```python
from build123d import *

# Parameters (mm, degrees)
BOSS_EXTRUDE1_DEPTH = 38.1
CUT_EXTRUDE1_DEPTH  = 98.457965419
SHELL1_START        = -37.25333418
SHELL1_DEPTH        = 74.50666836
FILLET1_R           = 17.78
SKETCH3_W           = 12.7
SKETCH3_H           = 13.97
CUT_EXTRUDE2_DEPTH  = 2.54


# Read off the part's stored shape, not the designer's step: Shell1
with BuildPart() as part:
    # Sketch1 → Boss-Extrude1 (new, symmetric)
    with BuildSketch(Plane.XY):
        Polygon((-33.198119966, 25.4), (-33.198119966, -25.4), (33.198119966, -50.887128572), (33.198119966, -0.087128572), align=None)
    extrude(amount=BOSS_EXTRUDE1_DEPTH, both=True)

    # Sketch2 → Cut-Extrude1 (cut, through all)
    with BuildSketch(Plane.XY.offset(38.1)):
        Polygon((16.599059983, -44.515346429), (33.198119966, -33.107128572), (33.198119966, -50.887128572), align=None)
        Polygon((-16.599059983, 19.028217857), (-33.198119966, 25.4), (-33.198119966, 7.62), align=None)
    extrude(amount=-CUT_EXTRUDE1_DEPTH, mode=Mode.SUBTRACT)

    # Shell1 outline → Shell1 (cut)
    with BuildSketch(Plane.XY.offset(SHELL1_START)):
        Polygon((-32.351454146, 7.174547563), (-32.351454146, -24.818102704), (16.486612201, -43.565279915), (31.928119966, -32.952625656), (31.928119966, 0.400378753), (-15.639946381, 18.66004864), align=None)
    extrude(amount=SHELL1_DEPTH, mode=Mode.SUBTRACT)

    # Fillet1
    # the kernel refuses this fillet: 17.78 mm, written as the material it adds along each edge
    with BuildSketch(Plane(origin=(-14.571454146, -12.59824726, -19.47333418), x_dir=(-1, 0, 0), z_dir=(0, 0, -1))) as fillet1_piece_1_section:
        Polygon((0, 0), (FILLET1_R * 1.02, 0), (FILLET1_R * 1.02, -FILLET1_R * 0.701026577777), (FILLET1_R * 0.365535308531, -FILLET1_R * 0.952252035029), align=None)
    fillet1_piece_1 = extrude(amount=FILLET1_R * 1.02, mode=Mode.PRIVATE)
    fillet1_piece_1 = fillet1_piece_1 - Plane(origin=(-14.571454146, -12.59824726, -19.47333418), x_dir=(0.8241261886205663, 0.5664062369269417, 0), z_dir=(0, 0, -1)) * Sphere(FILLET1_R, mode=Mode.PRIVATE)
    add(fillet1_piece_1)
    with BuildSketch(Plane(origin=(-14.571454146, -12.59824726, 19.47333418), x_dir=(-1, 0, 0), z_dir=(0, 0, 1))) as fillet1_piece_2_section:
        Polygon((0, 0), (FILLET1_R * 1.02, 0), (FILLET1_R * 1.02, FILLET1_R * 0.701026577777), (FILLET1_R * 0.365535308531, FILLET1_R * 0.952252035029), align=None)
    fillet1_piece_2 = extrude(amount=FILLET1_R * 1.02, mode=Mode.PRIVATE)
    fillet1_piece_2 = fillet1_piece_2 - Plane(origin=(-14.571454146, -12.59824726, 19.47333418), x_dir=(0.8241261886205663, 0.5664062369269417, 0), z_dir=(0, 0, 1)) * Sphere(FILLET1_R, mode=Mode.PRIVATE)
    add(fillet1_piece_2)
    with BuildSketch(Plane(origin=(-20.943236289, -29.197307243, -37.25333418), x_dir=(0.3583679495405225, 0.9335804264990358, 0), z_dir=(0.9335804264990358, -0.3583679495405224, 0))) as fillet1_piece_3_section:
        with BuildLine():
            CenterArc((FILLET1_R, FILLET1_R), FILLET1_R, 180, 90)
            Line((0, FILLET1_R), (0, 0))
            Line((0, 0), (FILLET1_R, 0))
        make_face()
    fillet1_piece_3 = extrude(amount=84.542794822, mode=Mode.PRIVATE)
    fillet1_piece_3 = split(fillet1_piece_3, bisect_by=Plane(origin=(31.928119966, -33.01813641, -33.386694553), z_dir=(-1, 0, 0)), keep=Keep.TOP, mode=Mode.PRIVATE)
    fillet1_piece_3 = split(fillet1_piece_3, bisect_by=Plane(origin=(10.612775853, -47.602255791, -33.386694553), z_dir=(-0.5664062369254325, 0.8241261886216036, 0)), keep=Keep.TOP, mode=Mode.PRIVATE)
    add(fillet1_piece_3)
    with BuildSketch(Plane(origin=(31.928119966, -77.402625656, -37.25333418), x_dir=(-1, 0, 0), z_dir=(0, 1, 0))) as fillet1_piece_4_section:
        with BuildLine():
            CenterArc((FILLET1_R, FILLET1_R), FILLET1_R, 180, 90)
            Line((0, FILLET1_R), (0, 0))
            Line((0, 0), (FILLET1_R, 0))
        make_face()
    fillet1_piece_4 = extrude(amount=122.253004409, mode=Mode.PRIVATE)
    fillet1_piece_4 = split(fillet1_piece_4, bisect_by=Plane(origin=(33.987840467, -0.39027387, -33.467977185), z_dir=(-0.3583679495453051, -0.9335804264972, 0)), keep=Keep.TOP, mode=Mode.PRIVATE)
    fillet1_piece_4 = split(fillet1_piece_4, bisect_by=Plane(origin=(17.295340959, -43.875721799, -33.467977185), z_dir=(0.3583679495405224, 0.9335804264990358, 0)), keep=Keep.TOP, mode=Mode.PRIVATE)
    fillet1_piece_4 = split(fillet1_piece_4, bisect_by=Plane(origin=(36.497116542, -29.812441309, -33.467977185), z_dir=(-0.5664062369254325, 0.8241261886216036, 0)), keep=Keep.TOP, mode=Mode.PRIVATE)
    add(fillet1_piece_4)
    with BuildSketch(Plane(origin=(-32.351454146, 51.624547563, 37.25333418), x_dir=(1, 0, 0), z_dir=(0, -1, 0))) as fillet1_piece_5_section:
        with BuildLine():
            CenterArc((FILLET1_R, -FILLET1_R), FILLET1_R, 90, 90)
            Line((0, -FILLET1_R), (0, 0))
            Line((0, 0), (FILLET1_R, 0))
        make_face()
    fillet1_piece_5 = extrude(amount=64.222794823, mode=Mode.PRIVATE)
    fillet1_piece_5 = split(fillet1_piece_5, bisect_by=Plane(origin=(-19.793272657, 20.254361223, 33.481549938), z_dir=(-0.3583679495453051, -0.9335804264972, 0)), keep=Keep.TOP, mode=Mode.PRIVATE)
    fillet1_piece_5 = split(fillet1_piece_5, bisect_by=Plane(origin=(-33.346924572, 6.490379695, 33.481549938), z_dir=(0.5664062369446778, -0.8241261886083766, 0)), keep=Keep.TOP, mode=Mode.PRIVATE)
    add(fillet1_piece_5)
    with BuildSketch(Plane(origin=(-20.943236289, -29.197307243, 37.25333418), x_dir=(0.3583679495405225, 0.9335804264990358, 0), z_dir=(0.9335804264990358, -0.3583679495405224, 0))) as fillet1_piece_6_section:
        with BuildLine():
            CenterArc((FILLET1_R, -FILLET1_R), FILLET1_R, 90, 90)
            Line((0, -FILLET1_R), (0, 0))
            Line((0, 0), (FILLET1_R, 0))
        make_face()
    fillet1_piece_6 = extrude(amount=84.542794822, mode=Mode.PRIVATE)
    fillet1_piece_6 = split(fillet1_piece_6, bisect_by=Plane(origin=(31.928119966, -33.01813641, 33.386694553), z_dir=(-1, 0, 0)), keep=Keep.TOP, mode=Mode.PRIVATE)
    fillet1_piece_6 = split(fillet1_piece_6, bisect_by=Plane(origin=(10.612775853, -47.602255791, 33.386694553), z_dir=(-0.5664062369254325, 0.8241261886216036, 0)), keep=Keep.TOP, mode=Mode.PRIVATE)
    add(fillet1_piece_6)
    with BuildSketch(Plane(origin=(31.928119966, -77.402625656, 37.25333418), x_dir=(-1, 0, 0), z_dir=(0, 1, 0))) as fillet1_piece_7_section:
        with BuildLine():
            CenterArc((FILLET1_R, -FILLET1_R), FILLET1_R, 90, 90)
            Line((0, -FILLET1_R), (0, 0))
            Line((0, 0), (FILLET1_R, 0))
        make_face()
    fillet1_piece_7 = extrude(amount=122.253004409, mode=Mode.PRIVATE)
    fillet1_piece_7 = split(fillet1_piece_7, bisect_by=Plane(origin=(33.987840467, -0.39027387, 33.467977185), z_dir=(-0.3583679495453051, -0.9335804264972, 0)), keep=Keep.TOP, mode=Mode.PRIVATE)
    fillet1_piece_7 = split(fillet1_piece_7, bisect_by=Plane(origin=(17.295340959, -43.875721799, 33.467977185), z_dir=(0.3583679495405224, 0.9335804264990358, 0)), keep=Keep.TOP, mode=Mode.PRIVATE)
    fillet1_piece_7 = split(fillet1_piece_7, bisect_by=Plane(origin=(36.497116542, -29.812441309, 33.467977185), z_dir=(-0.5664062369254325, 0.8241261886216036, 0)), keep=Keep.TOP, mode=Mode.PRIVATE)
    add(fillet1_piece_7)
    with BuildSketch(Plane(origin=(-32.351454146, -24.818102704, -19.47333418), x_dir=(0, 1, 0), z_dir=(0, 0, 1))) as fillet1_piece_8:
        with BuildLine():
            CenterArc((FILLET1_R * 0.687280958605, -FILLET1_R), FILLET1_R, 90, 69)
            Line((-FILLET1_R * 0.246299467894, -FILLET1_R * 0.641632050459), (0, 0))
            Line((0, 0), (FILLET1_R * 0.687280958605, 0))
        make_face()
    extrude(amount=38.94666836)
    with BuildSketch(Plane(origin=(-32.351454146, 51.624547563, -37.25333418), x_dir=(1, 0, 0), z_dir=(0, -1, 0))) as fillet1_piece_9_section:
        with BuildLine():
            CenterArc((FILLET1_R, FILLET1_R), FILLET1_R, 180, 90)
            Line((0, FILLET1_R), (0, 0))
            Line((0, 0), (FILLET1_R, 0))
        make_face()
    fillet1_piece_9 = extrude(amount=64.222794823, mode=Mode.PRIVATE)
    fillet1_piece_9 = split(fillet1_piece_9, bisect_by=Plane(origin=(-19.793272657, 20.254361223, -33.481549938), z_dir=(-0.3583679495453051, -0.9335804264972, 0)), keep=Keep.TOP, mode=Mode.PRIVATE)
    fillet1_piece_9 = split(fillet1_piece_9, bisect_by=Plane(origin=(-33.346924572, 6.490379695, -33.481549938), z_dir=(0.5664062369446778, -0.8241261886083766, 0)), keep=Keep.TOP, mode=Mode.PRIVATE)
    add(fillet1_piece_9)
    with BuildSketch(Plane(origin=(-32.351454146, 7.174547563, -37.25333418), x_dir=(0.8241261886083765, 0.5664062369446778, 0), z_dir=(0, 0, 1)), Plane(origin=(16.486612201, -43.565279915, -37.25333418), x_dir=(-0.933580426499036, 0.3583679495405219, 0), z_dir=(0, 0, 1))) as fillet1_piece_10:
        with BuildLine():
            CenterArc((FILLET1_R * 0.526125451477, -FILLET1_R), FILLET1_R, 90, 55.499999999)
            Line((-FILLET1_R * 0.298000737132, -FILLET1_R * 0.433593763055), (0, 0))
            Line((0, 0), (FILLET1_R * 0.526125451477, 0))
        make_face()
    extrude(amount=74.50666836)
    with BuildSketch(Plane(origin=(31.928119966, -32.952625656, -37.25333418), x_dir=(0, 1, 0), z_dir=(0, 0, 1))) as fillet1_piece_11:
        with BuildLine():
            CenterArc((FILLET1_R * 0.526125451492, FILLET1_R), FILLET1_R, 214.5, 55.5)
            Line((-FILLET1_R * 0.29800073713, FILLET1_R * 0.433593763075), (0, 0))
            Line((0, 0), (FILLET1_R * 0.526125451492, 0))
        make_face()
    extrude(amount=74.50666836)

    # Sketch3 → Cut-Extrude2 (cut)
    with BuildSketch(Plane(origin=(33.198119966, 0, 0), x_dir=(0, 0, -1), z_dir=(1, 0, 0))):
        with Locations((0, -5.802128572)):
            Rectangle(SKETCH3_W, SKETCH3_H)
    extrude(amount=-CUT_EXTRUDE2_DEPTH, mode=Mode.SUBTRACT)


solid = part.part
```
The model under review builds one solid part; all positions refer to its coordinate system, in mm. A direction names the side the tool comes from. Give positions to 0.01 mm unless a question says otherwise; leave off trailing zeros. Loops run counter-clockwise (first coordinate to the right, second up) from the corner with the lowest first, then second, coordinate; pieces in that order, holes last. Notation, with made-up numbers: (39, 88) - (88, 88) arc R16 ccw to (88, 118) - close; hole circle Ø7 at (11.25, 17.25). An arc over 180 degrees is marked (long way). Answer as a JSON object with one key per item and string values.
Q1. Add section C-C on x = 29. State the section outline as (y, z) points.
Worked out:
{"outline": "(-35.99, -38.1) - (1.52, -38.1) - (1.52, -29.25) - (-33.37, -29.25) - (-33.37, 29.25) - (1.52, 29.25) - (1.52, 38.1) - (-35.99, 38.1) - close"}
Q2. Add section A-A on y = -11.5. State the section outline as (x, z) points, plus the area to 3 significant figures.
Worked out:
{"outline": "(-33.2, -38.1) - (33.2, -38.1) - (33.2, -6.35) - (31.93, -6.35) - (31.93, -19.47) arc R17.78 cw to (14.15, -37.25) - (-14.57, -37.25) arc R17.78 cw to (-32.35, -19.47) - (-32.35, 19.47) arc R17.78 cw to (-14.57, 37.25) - (14.15, 37.25) arc R17.78 cw to (31.93, 19.47) - (31.93, 6.35) - (33.2, 6.35) - (33.2, 38.1) - (-33.2, 38.1) - close", "area": "525 mm^2"}
Q3. To check wall thickness, follow line 1 along Z through (x, y) = (-10, -12.5); line 2 along Z through (x, y) = (15.5, -20.5); line 3 along X through (y, z) = (-12, 15). State the ranges of each line that lie inside material, in increasing order.
Worked out:
{"line 1": "z = -38.1 to -37.25, 37.25 to 38.1", "line 2": "z = -38.1 to -37.2, 37.2 to 38.1", "line 3": "x = -33.2 to -32.35, 31.93 to 33.2"}
Q4. Insertion check: pin 1 (6 mm diameter, centred on x = 3, z = -14, fed in from +Y); pin 2 (4 mm diameter, centred on x = 4, z = -7, fed in from -Y); pin 3 (4 mm diameter, centred on y = 9.5, z = 6, fed in from -X); pin 4 (0.6 mm diameter, centred on x = 32, z = 1.5, fed in from +Y). Each pin has a flat end and moves straight along its axis. Give the tip position at first contact, or say it passes through.
Worked out:
{"pin 1": "stops at y = -37.24", "pin 2": "stops at y = -40.45", "pin 3": "stops at x = -33.2", "pin 4": "stops at y = -12.79"}
Q5. For faces 1 (the flat face through (-20.08, 15.61, -0.52)), 2 (the flat face through (-25.015, 13.244, 0.533)), 3 (the flat face through (0, -12, 38.1)), 4 (the cylindrical face through (26.858, -15.835, -31.907)), 5 (the cylindrical face through (-29.309, -22.545, -0.273)), list the 3-axis set-ups (+Z, -Z, +X, -X, +Y, -Y) from which the entire face can be reached by the end or side of a thin tool; tool diameter is ignored.
Worked out:
{"face 1": "+X", "face 2": "+Z, -Z, -X, +Y", "face 3": "+Z, +X, -X, +Y, -Y", "face 4": "+Y", "face 5": "none"}
Q6. Mouldability with a two-part tool opening along X and no side actions: class faces 6 (the flat face through (24.782, -38.891, 0.533)), 7 (the flat face through (-8.648, -34.824, 0.533)), 8 (the cylindrical face through (-2.84, -30.42, 32.18)) as +X half, -X half, draft (parallel to the pull), parting line (faces both ways), or undercut.
Worked out:
{"face 6": "+X half", "face 7": "-X half", "face 8": "undercut"}
